Here's how the part is built. I have some questions about the finished solid (model axes, mm). Face numbers are marked on the shaded views. A direction names the side the tool comes from. Give positions to 0.01 mm unless a question says otherwise; leave off trailing zeros. Loops run counter-clockwise (first coordinate to the right, second up) from the corner with the lowest first, then second, coordinate; pieces in that order, holes last.
Q1. Thinking about a two-plate mould opening in Z: for the marked faces 4, 5 and 6, which applies, pulls with the +Z half, pulls with the -Z half, needs draft (parallel to the pull), parting line crosses it, or undercut?
Q2. Suppose I cut it at C-C (z = 32.5). List the corners of the cut face in (x, y) for me.
Q3. I'm going to push flat-ended pins straight in: P1, Ø2, axis at x = 43, z = 37.5, coming from the +Y side; P2, Ø5, axis at x = 69, y = -6, coming from the -Z side; P3, Ø8, axis at x = 95, y = -7, coming from the +Z side. Where does each tip first touch, or does it pass through?
Q4. Suppose I cut it at B-B (x = 68). List the corners of the cut face in (y, z) for me, and give its area (3 significant figures).
Q5. I need wall thicknesses on probe 1 along Y at (x, z) = (95, 83); probe 2 along Y at (x, z) = (32.5, 79); probe 3 along Z at (x, y) = (75, -3.75). Which ranges of each line are inside material? Lowest first, please.
Q6. Suppose I cut it at D-D (x = 95). List the corners of the cut face in (y, z) for me.
Q7. Suppose I cut it at A-A (y = -5). List the corners of the cut face in (x, z) for me.
Q8. For the marked faces 1, 2 and 3, which set-ups out of +Z, -Z, +X, -X, +Y, -Y let a thin tool reach every point of the face, with its end or its side?
```python
from build123d import *

# Parameters (mm, degrees)
F1_DEPTH        = 10
F2_R            = 10
F4_DEPTH        = 10.001
F5_R            = 5
F6_W            = 75
F6_H            = 10
F7_DEPTH        = 10
F9_DEPTH        = 20.001
F11_D           = 6.6
F11_DEPTH       = 20
F11_CBORE_D     = 15
F11_CBORE_DEPTH = 6


with BuildPart() as f1:
    # F0 (on Front) → F1 (new body)
    with BuildSketch(Plane.XZ):
        Polygon((0, 95), (0, 0), (50, 0), (50, 20), (100, 20), (100, 95), align=None)
    extrude(amount=F1_DEPTH)

    # F2
    f2_edges = [f1.edges().sort_by_distance(p)[0] for p in [
        (100, -5, 20),
    ]]
    fillet(f2_edges, radius=F2_R)

    # F3 (on face) → F4 (cut, through all)
    with BuildSketch(Plane.XZ.offset(10)):
        with BuildLine():
            ThreePointArc((12.5, 12.5), (14.330583, 8.080583), (18.75, 6.25))
            Line((18.75, 6.25), (31.25, 6.25))
            ThreePointArc((31.25, 6.25), (35.669417, 8.080583), (37.5, 12.5))
            ThreePointArc((37.5, 12.5), (35.669417, 16.919417), (31.25, 18.75))
            Line((31.25, 18.75), (18.75, 18.75))
            ThreePointArc((18.75, 18.75), (14.330583, 16.919417), (12.5, 12.5))
        make_face()
    extrude(amount=-F4_DEPTH, mode=Mode.SUBTRACT)

    # F5
    f5_edges = [f1.edges().sort_by_distance(p)[0] for p in [
        (50, -5, 20),
        (50, -5, 0),
        (0, -5, 0),
        (0, -5, 95),
    ]]
    fillet(f5_edges, radius=F5_R)

    # F6 (on face) → F7 (join)
    with BuildSketch(Plane(origin=(0, 0, 0), x_dir=(-1, 0, 0), z_dir=(0, 1, 0))):
        with Locations((-37.5, 30)):
            Rectangle(F6_W, F6_H)
    extrude(amount=F7_DEPTH)

    # F8 (on face) → F9 (cut, through all)
    with BuildSketch(Plane.XZ.offset(10)):
        with BuildLine():
            Line((100, 75), (89.96663, 75))
            ThreePointArc((89.96663, 75), (60, 74), (89.96663, 73))
            Line((89.96663, 73), (100, 73))
            Line((100, 73), (100, 75))
        make_face()
    extrude(amount=-F9_DEPTH, mode=Mode.SUBTRACT)

    # F11
    with Locations(Plane.XY.offset(95)):
        with Locations((95, -5)):
            CounterBoreHole(F11_D / 2, F11_CBORE_D / 2, F11_CBORE_DEPTH, depth=F11_DEPTH)


solid = f1.part
```
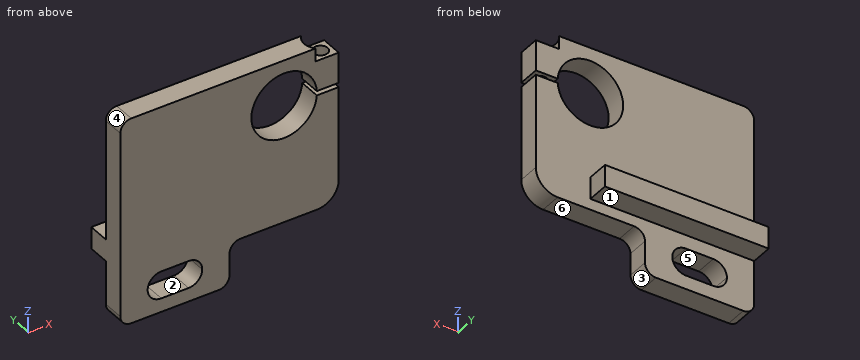
Solutions:
1. face 4: pulls with the +Z half
1. face 5: undercut
1. face 6: pulls with the -Z half
2. outline: (0, -10) - (100, -10) - (100, 0) - (75, 0) - (75, 10) - (0, 10) - close
3. P1: stops at y = 0
3. P2: stops at z = 20
3. P3: stops at z = 89
4. outline: (-10, 20) - (0, 20) - (0, 25) - (10, 25) - (10, 35) - (0, 35) - (0, 60.73) - (-10, 60.73) - close; (-10, 87.27) - (0, 87.27) - (0, 95) - (-10, 95) - close
4. area: 585 mm2
5. probe 1: y = -10 to -8.3, -1.7 to 0
5. probe 2: y = -10 to 0
5. probe 3: z = 20 to 59, 89 to 95
6. outline: (-10, 21.34) - (0, 21.34) - (0, 73) - (-10, 73) - close; (-10, 75) - (-8.3, 75) - (-8.3, 89) - (-10, 89) - close; (-1.7, 75) - (0, 75) - (0, 89) - (-1.7, 89) - close
7. outline: (0, 5) arc R5 ccw to (5, 0) - (45, 0) arc R5 ccw to (50, 5) - (50, 15) arc R5 cw to (55, 20) - (90, 20) arc R10 ccw to (100, 30) - (100, 73) - (89.97, 73) arc R15 cw (long way) to (89.97, 75) - (91.7, 75) - (91.7, 89) - (87.5, 89) - (87.5, 95) - (5, 95) arc R5 ccw to (0, 90) - close; (98.3, 75) - (100, 75) - (100, 89) - (98.3, 89) - close; hole (12.5, 12.5) arc R6.25 ccw to (18.75, 6.25) - (31.25, 6.25) arc R6.25 ccw to (37.5, 12.5) arc R6.25 ccw to (31.25, 18.75) - (18.75, 18.75) arc R6.25 ccw to start
8. face 1: -Z, +X, -X, +Y
8. face 2: +Y, -Y
8. face 3: -Z, +X, +Y, -Y
